Source: three-view drawing plus pictorial views. Frame: mm from the lowest corner of the part. A direction names the side the tool comes from. Give positions to 0.01 mm unless a question says otherwise; leave off trailing zeros. Loops run counter-clockwise (first coordinate to the right, second up) from the corner with the lowest first, then second, coordinate; pieces in that order, holes last. Notation, with made-up numbers: M 55,-15.5 L 94,-15.5 A30 cw 94,18.5 Z; hole C 46.5,73.5 d5. An arc over 180 degrees is marked long. Put each result on its own line as item: value. Start each with the question number.
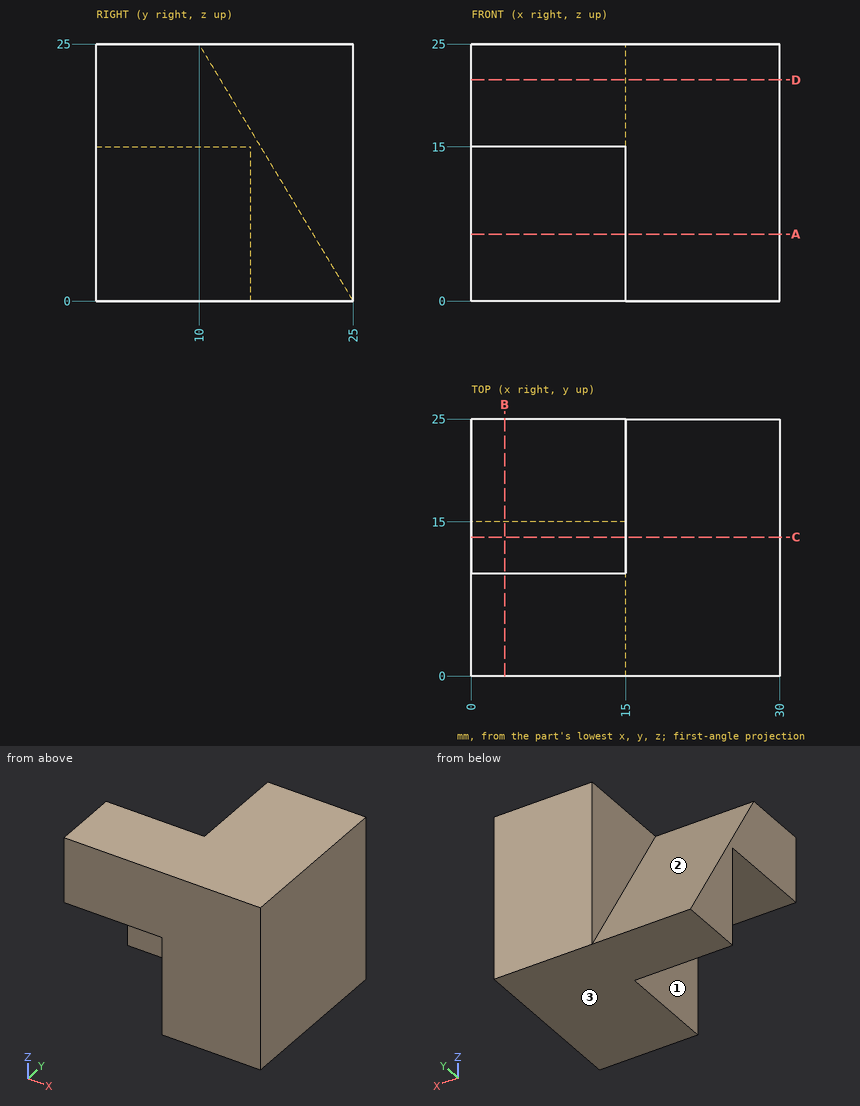
1. Section C-C, the plane y = 13.5. Output: boundary loops of the cut face in (x, z), plus the area to 4 significant figures.
2. Section A-A, the plane z = 6.5. Output: boundary loops of the cut face in (x, y).
3. Contact query for flat-ended pins moving along their axis: pin 1 (1.5 mm diameter, centred on x = 4, y = 13.5, fed in from -Z); pin 2 (4.5 mm diameter, centred on x = 7.5, z = 9.5, fed in from -Y); pin 3 (7.5 mm diameter, centred on y = 7.5, z = 5.5, fed in from -X). Output: stop coordinate, or through.
4. Set-up query: the marked faces 1, 2 and 3. Return all of +Z, -Z, +X, -X, +Y, -Y with unobstructed straight access to the full face (end or side cutting, diameter ignored); none if empty.
5. Ray query, line 1 (Z direction, x = 5.5, y = 2.5); line 2 (X direction, y = 2, z = 12.75); line 3 (Z direction, x = 11.75, y = 14.5). Return the intervals inside material, ascending.
6. Section B-B, the plane x = 3.25. Output: boundary loops of the cut face in (y, z), plus the area to 4 significant figures.
7. Section D-D, the plane z = 21.5. Output: boundary loops of the cut face in (x, y), plus the area to 4 significant figures.
Results found:
1. outline: M 0,15 L 15,15 L 15,0 L 30,0 L 30,25 L 15,25 L 15,19.17 L 0,19.17 Z
1. area: 437.5 mm²
2. outline: M 0,15 L 15,15 L 15,0 L 30,0 L 30,25 L 15,25 L 15,21.1 L 0,21.1 Z
3. pin 1: z = 15
3. pin 2: y = 15
3. pin 3: x = 15
4. face 1: -Z, -X, -Y
4. face 2: +Z, -X, +Y
4. face 3: -Z, +X, -X, +Y, -Y
5. line 1: 15 to 25
5. line 2: 15 to 30
5. line 3: 15 to 17.5
6. outline: M 0,15 L 15,15 L 15,0 L 25,0 L 10,25 L 0,25 Z
6. area: 212.5 mm²
7. outline: M 0,0 L 30,0 L 30,25 L 15,25 L 15,12.1 L 0,12.1 Z
7. area: 556.5 mm²
